```python
from build123d import *

# Parameters (mm, degrees)
F2_R          = 20
F3_DEPTH      = 2
F4_W          = 15.1418782771
F4_H          = 14.9113200605
F5_DEPTH      = 25
F5_DEPTH_BACK = 25


with BuildPart() as f1:
    # F0 (on Front) → F1 (revolve)
    with BuildSketch(Plane.XZ):
        Polygon((0, 40), (0, 0), (20, 0), align=None)
    revolve(axis=Axis((0, 0, 20), (0, 0, 1)))

    # F2 (on Top) → F3 (join)
    with BuildSketch(Plane.XY):
        Circle(F2_R)
    extrude(amount=F3_DEPTH)

    # F4 (on Front) → F5 (cut, two sides)
    with BuildSketch(Plane.XZ) as f5_sk:
        with Locations((0.5040215328, 38.1232108921)):
            Rectangle(F4_W, F4_H)
    extrude(amount=-F5_DEPTH, mode=Mode.SUBTRACT)
    extrude(f5_sk.sketch, amount=F5_DEPTH_BACK, mode=Mode.SUBTRACT)


solid = f1.part
```
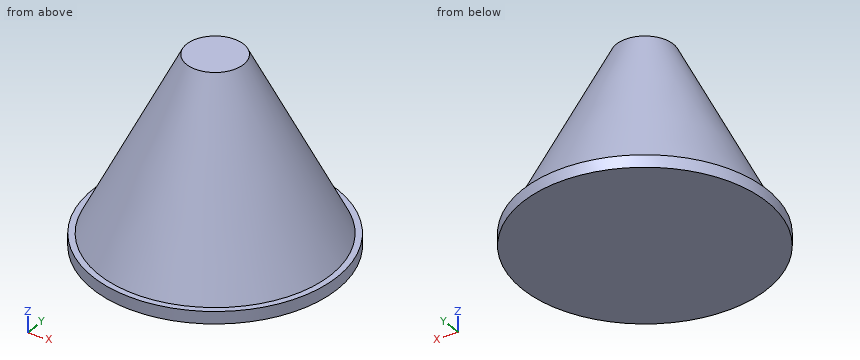
Part model, mm, in its own coordinate system. Round coordinates to 2 decimals unless told otherwise and drop trailing zeros. Loops run counter-clockwise (first coordinate to the right, second up) from the corner with the lowest first, then second, coordinate; pieces in that order, holes last.
Item 1: Cut at C-C, the plane z = 8. Give the cut face in (x, y).
Item 2: Cut at A-A, the plane y = 0. Give the cut face in (x, z).
Item 3: Cut at D-D, the plane z = 26.5. Give the cut face in (x, y).
Item 4: Drill centre lines: line 1 (Y direction, x = 5.5, z = 23); line 2 (Z direction, x = 8, y = 17); line 3 (Z direction, x = -5, y = -4). Where is each one in solid material? Low to high.
Item 5: Drop flat-ended pins along their axis: P1, Ø1, axis at y = -1, z = 21, coming from the +X side; P2, Ø8, axis at x = 15.5, y = 0.5, coming from the +Z side; P3, Ø5, axis at y = 5, z = 10.5, coming from the +X side. Give the stop position or say it passes through.
A:
1. outline: circle Ø32 at (0, 0)
2. outline: (-20, 0) - (20, 0) - (20, 2) - (19, 2) - (4.67, 30.67) - (-4.67, 30.67) - (-19, 2) - (-20, 2) - close
3. outline: circle Ø13.5 at (0, 0)
4. line 1: y = -6.48 to 6.48
4. line 2: z = 0 to 2.42
4. line 3: z = 0 to 27.19
5. P1: stops at x = 9.7
5. P2: stops at z = 16.98
5. P3: stops at x = 15.39
